Here's how the part is built. I have some questions about the finished solid (model axes, mm). A direction names the side the tool comes from. Coordinates: 2 decimals unless noted, no trailing zeros. Write each loop counter-clockwise with the first axis right and the second up, starting at its lowest first coordinate (ties: lowest second). Pieces come first, ordered by that corner, then holes.
(1) Imagine slicing it at C-C, the plane x = -8. List the corners of the cut face in (y, z) for me.
(2) Thinking about a two-plate mould opening in Y: for faces 4 (the cylindrical face through (1.336, 0.421, 54.108)), 5 (the cylindrical face through (-0.468, -3.562, 60.281)), 6 (the flat face through (-9, -6, 8.89)), which applies, released by +Y, released by -Y, zero draft, split by the parting line, or undercut?
(3) Imagine slicing it at A-A, the plane x = 0. List the corners of the cut face in (y, z) for me.
(4) Please list where these lines run through material, in increasing order: probe 1 along Y at (x, z) = (0, 53); probe 2 along Y at (x, z) = (0, 59.5); probe 3 along Z at (x, y) = (-3.25, 6.25).
(5) For pin 1 Ø12 at (x, z) = (4.5, 38.5) entering from -Y; pin 2 Ø1.5 at (y, z) = (9, 29.5) entering from -X; pin 3 Ø10 at (x, z) = (-9, 53) entering from -Y; pin 4 Ø2.5 at (x, y) = (0, 0) entering from +Z, each with a flat end and sliding along its axis, tell me the tip position at first contact or that it passes through.
(6) Which directions (+Z, -Z, +X, -X, +Y, -Y) give clear straight access to the entire face, cutting with the end or side of a thin tool? Please do faces 1 (the flat face through (3, -3, 0)), 2 (the cylindrical face through (-2.257, -10.164, 32.682)), 3 (the cylindrical face through (-0.468, 3.562, 21.914)).
```python
from build123d import *

# Parameters (mm, degrees)
F0_R     = 13.0362037077
F0_R_2   = 10.4116007046
F0_R_3   = 3.592976873
F1_DEPTH = 12.7
F2_DEPTH = 57.15
F3_DEPTH = 50.8
F4_DEPTH = 3.81
F5_DEPTH = 44.45
F6_R     = 1.4003561132
F7_DEPTH = 63.501


with BuildPart() as f1:
    # F0 (on Top) → F1 (new body)
    with BuildSketch(Plane.XY):
        Circle(F0_R)
        Circle(F0_R_2, mode=Mode.SUBTRACT)
        Circle(F0_R_2)
        Circle(F0_R_3, mode=Mode.SUBTRACT)
        Circle(F0_R_3)
    extrude(amount=F1_DEPTH)

    # F0 (on Top) → F2 (join)
    with BuildSketch(Plane.XY):
        Circle(F0_R_2)
        Circle(F0_R_3, mode=Mode.SUBTRACT)
    extrude(amount=F2_DEPTH)

    # F3 (add): a face of the model
    f3_faces = [f1.faces().sort_by_distance(p)[0] for p in [
        (0, 0, 12.7),
    ]]
    extrude(f3_faces, amount=F3_DEPTH)

    # F4 (cut): a face of the model
    f4_faces = [f1.faces().sort_by_distance(p)[0] for p in [
        (-12.667484186, 0, 12.7),
    ]]
    extrude(f4_faces, amount=-F4_DEPTH, mode=Mode.SUBTRACT)

    # F0 (on Top) → F5 (cut)
    with BuildSketch(Plane.XY):
        Circle(F0_R_3)
    extrude(amount=F5_DEPTH, mode=Mode.SUBTRACT)

    # F6 (on face) → F7 (cut, through all)
    with BuildSketch(Plane.XY.offset(63.5)):
        Circle(F6_R)
    extrude(amount=-F7_DEPTH, mode=Mode.SUBTRACT)


solid = f1.part
```
Recorded:
1. outline: (-10.29, 0) - (10.29, 0) - (10.29, 8.89) - (6.66, 8.89) - (6.66, 57.15) - (-6.66, 57.15) - (-6.66, 8.89) - (-10.29, 8.89) - close
2. face 4: undercut
2. face 5: split by the parting line
2. face 6: zero draft
3. outline: (-13.04, 0) - (-3.59, 0) - (-3.59, 44.45) - (-1.4, 44.45) - (-1.4, 63.5) - (-3.59, 63.5) - (-3.59, 57.15) - (-10.41, 57.15) - (-10.41, 8.89) - (-13.04, 8.89) - close; (1.4, 44.45) - (3.59, 44.45) - (3.59, 0) - (13.04, 0) - (13.04, 8.89) - (10.41, 8.89) - (10.41, 57.15) - (3.59, 57.15) - (3.59, 63.5) - (1.4, 63.5) - close
4. probe 1: y = -10.41 to -1.4, 1.4 to 10.41
4. probe 2: y = -3.59 to -1.4, 1.4 to 3.59
4. probe 3: z = 0 to 57.15
5. pin 1: stops at y = -10.41
5. pin 2: stops at x = -6.35
5. pin 3: stops at y = -9.61
5. pin 4: passes through
6. face 1: -Z, +X, -X, +Y, -Y
6. face 2: +Z
6. face 3: -Z
